Build history of the part. All positions in model axes, mm. A direction names the side the tool comes from. Round coordinates to 2 decimals unless told otherwise and drop trailing zeros. Loops run counter-clockwise (first coordinate to the right, second up) from the corner with the lowest first, then second, coordinate; pieces in that order, holes last. Notation, with made-up numbers: (-9, 76.25) - (42, 76.25) arc R22 cw to (42, 103.25) - close; hole circle Ø3 at (-35, 84.25). An arc over 180 degrees is marked (long way). One line per question, with ' | ' between items. Start each with the question number.
from build123d import *

# Parameters (mm, degrees)
F0_R     = 8.25
F0_R_2   = 3
F0_R_3   = 1
F0_R_4   = 4
F1_DEPTH = 5
F2_DEPTH = 2


with BuildPart() as f1:
    # F0 (on Top) → F1 (new body)
    with BuildSketch(Plane.XY):
        with BuildLine():
            Line((-6, 18.919781), (-6, 8.919781))
            ThreePointArc((-6, 8.919781), (-8.736982, 6.263198), (-10.374039, 2.818123))
            ThreePointArc((-10.374039, 2.818123), (-10.655595, 1.421545), (-10.75, 0))
            ThreePointArc((-10.75, 0), (0, -10.75), (10.75, 0))
            ThreePointArc((10.75, 0), (10.655595, 1.421545), (10.374039, 2.818123))
            ThreePointArc((10.374039, 2.818123), (8.736982, 6.263198), (6, 8.919781))
            Line((6, 8.919781), (6, 18.919781))
            Line((6, 18.919781), (6, 40))
            ThreePointArc((6, 40), (0, 46), (-6, 40))
            Line((-6, 40), (-6, 18.919781))
        make_face()
        Circle(F0_R, mode=Mode.SUBTRACT)
        with Locations((0, 40)):
            Circle(F0_R_2, mode=Mode.SUBTRACT)
        Circle(F0_R)
        with Locations((-6, 0)):
            Circle(F0_R_3, mode=Mode.SUBTRACT)
        with Locations((-4.242641, -4.242641)):
            Circle(F0_R_3, mode=Mode.SUBTRACT)
        with Locations((-4.242641, 4.242641)):
            Circle(F0_R_3, mode=Mode.SUBTRACT)
        with Locations((0, -6)):
            Circle(F0_R_3, mode=Mode.SUBTRACT)
        with Locations((4.242641, -4.242641)):
            Circle(F0_R_3, mode=Mode.SUBTRACT)
        Circle(F0_R_4, mode=Mode.SUBTRACT)
        with Locations((4.242641, 4.242641)):
            Circle(F0_R_3, mode=Mode.SUBTRACT)
        with Locations((6, 0)):
            Circle(F0_R_3, mode=Mode.SUBTRACT)
        with Locations((0, 6)):
            Circle(F0_R_3, mode=Mode.SUBTRACT)
        with BuildLine():
            ThreePointArc((-10.374039, 2.818123), (-8.736982, 6.263198), (-6, 8.919781))
            Line((-6, 8.919781), (-6, 18.919781))
            Line((-6, 18.919781), (-10.374039, 2.818123))
        make_face()
        with BuildLine():
            ThreePointArc((6, 8.919781), (8.736982, 6.263198), (10.374039, 2.818123))
            Line((10.374039, 2.818123), (6, 18.919781))
            Line((6, 18.919781), (6, 8.919781))
        make_face()
    extrude(amount=F1_DEPTH)

    # F0 (on Top) → F2 (cut)
    with BuildSketch(Plane.XY):
        Circle(F0_R)
        with Locations((-6, 0)):
            Circle(F0_R_3, mode=Mode.SUBTRACT)
        with Locations((-4.242641, -4.242641)):
            Circle(F0_R_3, mode=Mode.SUBTRACT)
        with Locations((-4.242641, 4.242641)):
            Circle(F0_R_3, mode=Mode.SUBTRACT)
        with Locations((0, -6)):
            Circle(F0_R_3, mode=Mode.SUBTRACT)
        with Locations((4.242641, -4.242641)):
            Circle(F0_R_3, mode=Mode.SUBTRACT)
        Circle(F0_R_4, mode=Mode.SUBTRACT)
        with Locations((4.242641, 4.242641)):
            Circle(F0_R_3, mode=Mode.SUBTRACT)
        with Locations((6, 0)):
            Circle(F0_R_3, mode=Mode.SUBTRACT)
        with Locations((0, 6)):
            Circle(F0_R_3, mode=Mode.SUBTRACT)
    extrude(amount=F2_DEPTH, mode=Mode.SUBTRACT)


solid = f1.part
1) Wall check: line 1 (Y direction, x = 0, z = 3.4); line 2 (Y direction, x = 0, z = 1.3); line 3 (Y direction, x = 2.25, z = 4.1). Give the ranges that are in metal, low to high. Write a range as [from, to].
2) Drop flat-ended pins along their axis: pin 1 (7 mm diameter, centred on x = 0, y = 0, fed in from +Z); pin 2 (2 mm diameter, centred on y = 21.5, z = 2, fed in from -X); pin 3 (2.5 mm diameter, centred on x = -4.24, y = -4.24, fed in from -Z); pin 4 (3 mm diameter, centred on y = 10.5, z = 0.5, fed in from +X). Give the stop position or say it passes through.
3) Saw through at C-C on x = -2.5. Write the cut outline in (y, z).
4) Saw through at A-A on x = 0. Write the cut outline in (y, z).
5) Saw through at D-D on x = -6.5. Write the cut outline in (y, z).
6) Saw through at B-B on z = 0.85. Write the cut outline in (x, y), and give its area (3 significant figures).
7) Tool access for faces 5 (the cylindrical face through (0, 43, 2)), 6 (the flat face through (-6, 30, 2)), 7 (the flat face through (6, 29, 2)), 8 (the cylindrical face through (7.62, -3.16, 0.99)): list every direction of +Z, -Z, +X, -X, +Y, -Y with a clear straight run to the whole face (end or side of a thin tool).
8) Two-plate mould, pull along X, no slides. Class faces 1 (the flat face through (0, 18, 0)), 2 (the flat face through (8.218, 10.756, 2.465)), 3 (the cylindrical face through (-5.24, -4.2, 3.48)), 4 (the cylindrical face through (0, 46, 2)): +X half, -X half, draft (parallel to the pull), parting line (faces both ways), or undercut.
Answer key:
1) line 1: [-10.75, -7], [-5, -4], [4, 5], [7, 37], [43, 46] | line 2: [-10.75, -8.25], [8.25, 37], [43, 46] | line 3: [-10.51, -3.31], [3.31, 38.02], [41.98, 45.56]
2) pin 1: through | pin 2: x = -6 | pin 3: z = 2 | pin 4: x = 8.69
3) outline: (-10.46, 0) - (-7.86, 0) - (-7.86, 2) - (-3.12, 2) - (-3.12, 5) - (-10.46, 5) - close; (3.12, 2) - (7.86, 2) - (7.86, 0) - (38.34, 0) - (38.34, 5) - (3.12, 5) - close; (41.66, 0) - (45.45, 0) - (45.45, 5) - (41.66, 5) - close
4) outline: (-10.75, 0) - (-8.25, 0) - (-8.25, 2) - (-7, 2) - (-7, 5) - (-10.75, 5) - close; (-5, 2) - (-4, 2) - (-4, 5) - (-5, 5) - close; (4, 2) - (5, 2) - (5, 5) - (4, 5) - close; (7, 2) - (8.25, 2) - (8.25, 0) - (37, 0) - (37, 5) - (7, 5) - close; (43, 0) - (46, 0) - (46, 5) - (43, 5) - close
5) outline: (-8.56, 0) - (-5.08, 0) - (-5.08, 2) - (-0.87, 2) - (-0.87, 5) - (-8.56, 5) - close; (0.87, 2) - (5.08, 2) - (5.08, 0) - (17.08, 0) - (17.08, 5) - (0.87, 5) - close
6) outline: (-10.75, 0) arc R10.75 ccw to (10.75, 0) arc R10.75 ccw to (10.37, 2.82) - (6, 18.92) - (6, 40) arc R6 ccw to (-6, 40) - (-6, 18.92) - (-10.37, 2.82) arc R10.75 ccw to start; hole circle Ø16.5 at (0, 0); hole circle Ø6 at (0, 40) | area: 572 mm²
7) face 5: +Z, -Z | face 6: +Z, -Z, -X, +Y | face 7: +Z, -Z, +X, +Y | face 8: -Z
8) face 1: draft | face 2: +X half | face 3: undercut | face 4: parting line
